Geometry check sheet. Reference: the model listing, model coordinates, mm. Give positions to 0.01 mm unless a question says otherwise; leave off trailing zeros. Loops run counter-clockwise (first coordinate to the right, second up) from the corner with the lowest first, then second, coordinate; pieces in that order, holes last.
1. Release check for a two-part mould opening along Y. For faces 1 (the flat face through (0, 15.681, 0)), 2 (the cylindrical face through (-17.495, 16.847, -22.737)), 3 (the cylindrical face through (32.873, 11.056, 60.386)) record: +Y half, -Y half, draft (parallel to the pull), parting line (faces both ways), or undercut.
2. Cross-section at A-A, the plane z = -73. Record the cut outline in (x, y) (3 decimals), plus the area to 3 significant figures.
3. Cross-section at C-C, the plane z = -37.5. Record the cut outline in (x, y) (3 decimals), plus the area to 3 significant figures.
4. Go/stop test with a flat-tipped pin: pin 1 Ø19 at (x, z) = (13.5, 8.5) entering from -Y. Record where the tip stops, or that it passes through.
5. Material ranges on L1, parallel to Z at x = 5, y = 17.25; L2, parallel to X at y = 16.4, z = -13.5; L3, parallel to X at y = 8.5, z = 73 (3 decimals), recorded low to high.
6. Cross-section at B-B, the plane x = 17.3. Record the cut outline in (y, z), plus the area to 3 significant figures.
7. Cross-section at D-D, the plane z = -13.5. Record the cut outline in (x, y) (3 decimals).
from build123d import *

# Parameters (mm, degrees)
BOSS_EXTRUDE1_DEPTH   = 80
SKETCH2_W             = 8
SKETCH2_H             = 60
SKETCH2_W_2           = 29.5
CUT_EXTRUDE1_DEPTH    = 160
SKETCH3_R             = 1.5
CUT_EXTRUDE2_DEPTH    = 160
F_3_0MM_DOWEL_HOLE1_D = 3
LPATTERN1_COUNT       = 5
LPATTERN1_PITCH       = 14
F_3_0MM_DOWEL_HOLE2_D = 3
LPATTERN2_COUNT       = 5
LPATTERN2_PITCH       = 14


with BuildPart() as part:
    # Sketch1 → Boss-Extrude1 (new body, symmetric)
    with BuildSketch(Plane.XY):
        Polygon((-34, 17.981191673), (34, 17.981191673), (34, 5.281191673), (31.715, 5.281191673), (31.715, 15.681191673), (-31.715, 15.681191673), (-31.715, 5.281191673), (-34, 5.281191673), align=None)
    extrude(amount=BOSS_EXTRUDE1_DEPTH, both=True)

    # Sketch2 → Cut-Extrude1 (cut)
    with BuildSketch(Plane(origin=(0, 17.981191673, 0), x_dir=(1, 0, 0), z_dir=(0, 1, 0))):
        with Locations((-24, 46)):
            Rectangle(SKETCH2_W, SKETCH2_H)
        with Locations((0, 46)):
            Rectangle(SKETCH2_W_2, SKETCH2_H)
        with Locations((24, 46)):
            Rectangle(SKETCH2_W, SKETCH2_H)
        with Locations((24, -46)):
            Rectangle(SKETCH2_W, SKETCH2_H)
        with Locations((0, -46)):
            Rectangle(SKETCH2_W_2, SKETCH2_H)
        with Locations((-24, -46)):
            Rectangle(SKETCH2_W, SKETCH2_H)
    extrude(amount=-CUT_EXTRUDE1_DEPTH, mode=Mode.SUBTRACT)

    # Sketch3 → Cut-Extrude2 (cut)
    with BuildSketch(Plane(origin=(0, 17.981191673, 0), x_dir=(1, 0, 0), z_dir=(0, 1, 0))):
        with Locations((-17.3, 65.25)):
            Circle(SKETCH3_R)
        with Locations((-11, 13.5)):
            Circle(SKETCH3_R)
        with Locations((17.3, 65.25)):
            Circle(SKETCH3_R)
        with Locations((17.3, 43.25)):
            Circle(SKETCH3_R)
        with Locations((17.3, 21.25)):
            Circle(SKETCH3_R)
        with Locations((-17.3, 43.25)):
            Circle(SKETCH3_R)
        with Locations((-17.3, 21.25)):
            Circle(SKETCH3_R)
        with Locations((11, 13.5)):
            Circle(SKETCH3_R)
        with Locations((17.3, -65.25)):
            Circle(SKETCH3_R)
        with Locations((17.3, -43.25)):
            Circle(SKETCH3_R)
        with Locations((17.3, -21.25)):
            Circle(SKETCH3_R)
        with Locations((11, -13.5)):
            Circle(SKETCH3_R)
        with Locations((-11, -13.5)):
            Circle(SKETCH3_R)
        with Locations((-17.3, -21.25)):
            Circle(SKETCH3_R)
        with Locations((-17.3, -43.25)):
            Circle(SKETCH3_R)
        with Locations((-17.3, -65.25)):
            Circle(SKETCH3_R)
    extrude(amount=-CUT_EXTRUDE2_DEPTH, mode=Mode.SUBTRACT)

    # Ø3.0mm Dowel Hole1 (through all)
    with Locations(Plane(origin=(-34, 10.481191673, -73), x_dir=(0, 0, -1), z_dir=(-1, 0, 0))):
        with Locations((0, 0)):
            f_3_0mm_dowel_hole1 = Hole(F_3_0MM_DOWEL_HOLE1_D / 2)

    # LPattern1: Ø3.0mm Dowel Hole1 ×5
    with Locations(*[(0, 0, i * LPATTERN1_PITCH) for i in range(1, LPATTERN1_COUNT)]):
        add(f_3_0mm_dowel_hole1, mode=Mode.SUBTRACT)

    # Ø3.0mm Dowel Hole2 (through all)
    with Locations(Plane(origin=(-34, 10.481191673, 73), x_dir=(0, 0, -1), z_dir=(-1, 0, 0))):
        with Locations((0, 0)):
            f_3_0mm_dowel_hole2 = Hole(F_3_0MM_DOWEL_HOLE2_D / 2)

    # LPattern2: Ø3.0mm Dowel Hole2 ×5
    with Locations(*[(0, 0, -i * LPATTERN2_PITCH) for i in range(1, LPATTERN2_COUNT)]):
        add(f_3_0mm_dowel_hole2, mode=Mode.SUBTRACT)


solid = part.part
Result:
1. face 1: -Y half
1. face 2: draft
1. face 3: undercut
2. outline: (-34, 5.281) - (-31.715, 5.281) - (-31.715, 8.981) - (-34, 8.981) - close; (-34, 11.981) - (-31.715, 11.981) - (-31.715, 15.681) - (-28, 15.681) - (-28, 17.981) - (-34, 17.981) - close; (-20, 15.681) - (-14.75, 15.681) - (-14.75, 17.981) - (-20, 17.981) - close; (14.75, 15.681) - (20, 15.681) - (20, 17.981) - (14.75, 17.981) - close; (28, 15.681) - (31.715, 15.681) - (31.715, 11.981) - (34, 11.981) - (34, 17.981) - (28, 17.981) - close; (31.715, 5.281) - (34, 5.281) - (34, 8.981) - (31.715, 8.981) - close
2. area: 85.6 mm2
3. outline: (-34, 5.281) - (-31.715, 5.281) - (-31.715, 15.681) - (-28, 15.681) - (-28, 17.981) - (-34, 17.981) - close; (-20, 15.681) - (-14.75, 15.681) - (-14.75, 17.981) - (-20, 17.981) - close; (14.75, 15.681) - (20, 15.681) - (20, 17.981) - (14.75, 17.981) - close; (28, 15.681) - (31.715, 15.681) - (31.715, 5.281) - (34, 5.281) - (34, 17.981) - (28, 17.981) - close
3. area: 99.3 mm2
4. pin 1: stops at y = 15.68
5. L1: z = -80 to -76, -16 to 16, 76 to 80
5. L2: x = -34 to -12.5, -9.5 to 9.5, 12.5 to 34
5. L3: x = -34 to -31.715, 31.715 to 34
6. outline: (15.68, -80) - (17.98, -80) - (17.98, -66.75) - (15.68, -66.75) - close; (15.68, -63.75) - (17.98, -63.75) - (17.98, -44.75) - (15.68, -44.75) - close; (15.68, -41.75) - (17.98, -41.75) - (17.98, -22.75) - (15.68, -22.75) - close; (15.68, -19.75) - (17.98, -19.75) - (17.98, 19.75) - (15.68, 19.75) - close; (15.68, 22.75) - (17.98, 22.75) - (17.98, 41.75) - (15.68, 41.75) - close; (15.68, 44.75) - (17.98, 44.75) - (17.98, 63.75) - (15.68, 63.75) - close; (15.68, 66.75) - (17.98, 66.75) - (17.98, 80) - (15.68, 80) - close
6. area: 327 mm2
7. outline: (-34, 5.281) - (-31.715, 5.281) - (-31.715, 15.681) - (-12.5, 15.681) - (-12.5, 17.981) - (-34, 17.981) - close; (-9.5, 15.681) - (9.5, 15.681) - (9.5, 17.981) - (-9.5, 17.981) - close; (12.5, 15.681) - (31.715, 15.681) - (31.715, 5.281) - (34, 5.281) - (34, 17.981) - (12.5, 17.981) - close
